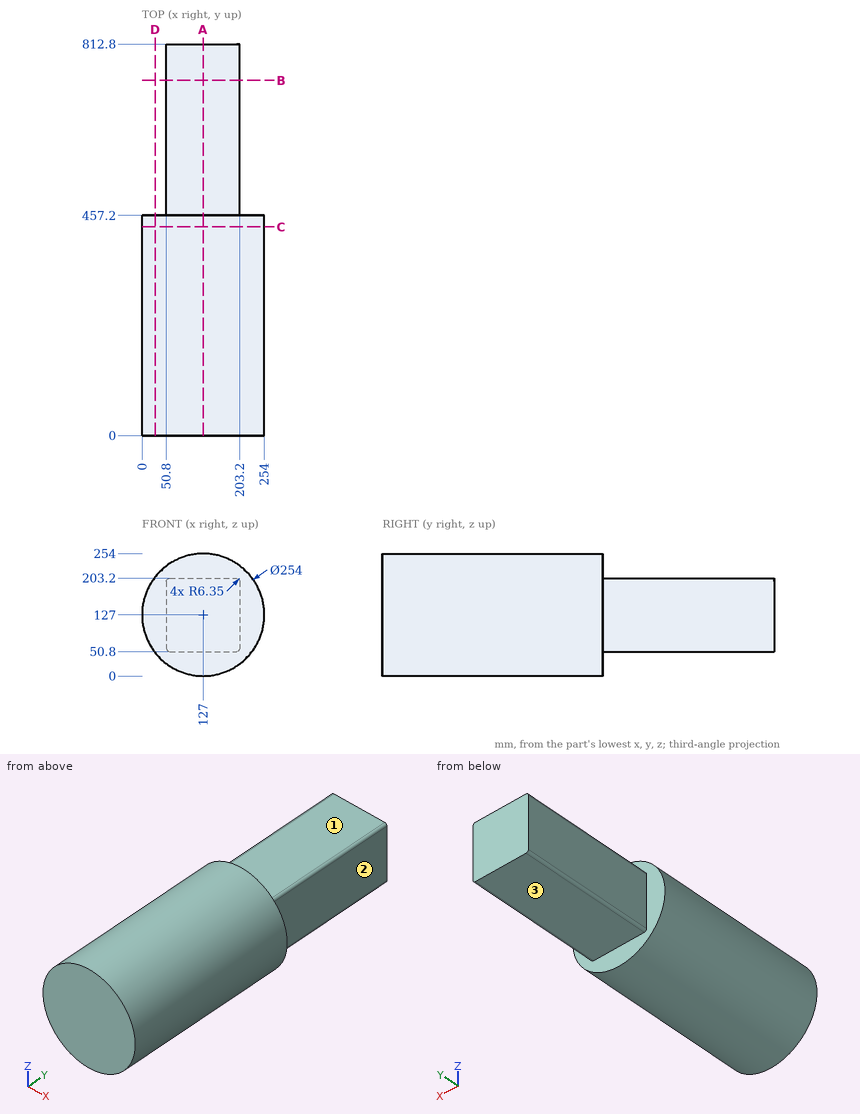
Part print with two shaded views. Sizes in mm from the minimum x, y, z corner. A direction names the side the tool comes from. Coordinates: 2 decimals unless noted, no trailing zeros. Write each loop counter-clockwise with the first axis right and the second up, starting at its lowest first coordinate (ties: lowest second). Pieces come first, ordered by that corner, then holes.
1. Band-saw the part on B-B, the plane y = 737.5. Give the cut face in (x, z), and give its area (3 significant figures).
Answer block:
outline: (50.8, 57.15) arc R6.35 ccw to (57.15, 50.8) - (196.85, 50.8) arc R6.35 ccw to (203.2, 57.15) - (203.2, 196.85) arc R6.35 ccw to (196.85, 203.2) - (57.15, 203.2) arc R6.35 ccw to (50.8, 196.85) - close
area: 23,200 mm2
2. Band-saw the part on D-D, the plane x = 27. Give the cut face in (y, z), and give its area (3 significant figures).
Answer block:
outline: (0, 48.71) - (457.2, 48.71) - (457.2, 205.29) - (0, 205.29) - close
area: 71,600 mm2
3. 3-axis set-ups, long thin cutter, end or side, ignore diameter. For the marked faces 1, 2 and 3: which of +Z, -Z, +X, -X, +Y, -Y reach the whole face in a straight line?
Answer block:
face 1: +Z, +X, -X, +Y
face 2: +Z, -Z, +X, +Y
face 3: -Z, +X, -X, +Y
4. Drill centre lines: probe 1 along Y at (x, z) = (57, 47); probe 2 along Z at (x, y) = (131, 539). Where is each one in solid material? Low to high.
Answer block:
probe 1: y = 0 to 457.2
probe 2: z = 50.8 to 203.2
5. Band-saw the part on A-A, the plane x = 127. Give the cut face in (y, z).
Answer block:
outline: (0, 0) - (457.2, 0) - (457.2, 50.8) - (812.8, 50.8) - (812.8, 203.2) - (457.2, 203.2) - (457.2, 254) - (0, 254) - close
6. Drop flat-ended pins along their axis: pin 1 (6 mm diameter, centred on x = 54.5, y = 688, fed in from +Z); pin 2 (6 mm diameter, centred on x = 140, y = 199.5, fed in from -Z); pin 3 (4 mm diameter, centred on x = 43, z = 110, fed in from -Y); pin 4 (1.5 mm diameter, centred on x = 165, y = 219, fed in from -Z). Give the stop position or say it passes through.
Answer block:
pin 1: stops at z = 203.2
pin 2: stops at z = 0.39
pin 3: stops at y = 0
pin 4: stops at z = 5.59
7. Band-saw the part on C-C, the plane y = 433. Give the cut face in (x, z).
Answer block:
outline: circle Ø254 at (127, 127)
